Verification items for this drawing (mm, ordinates from the low corner). Give positions to 0.01 mm unless a question says otherwise; leave off trailing zeros. Order: outer loops, then holes, each group sorted by start corner. A loop starts at its lowest first (then second) coordinate and runs counter-clockwise, first axis right, second up.
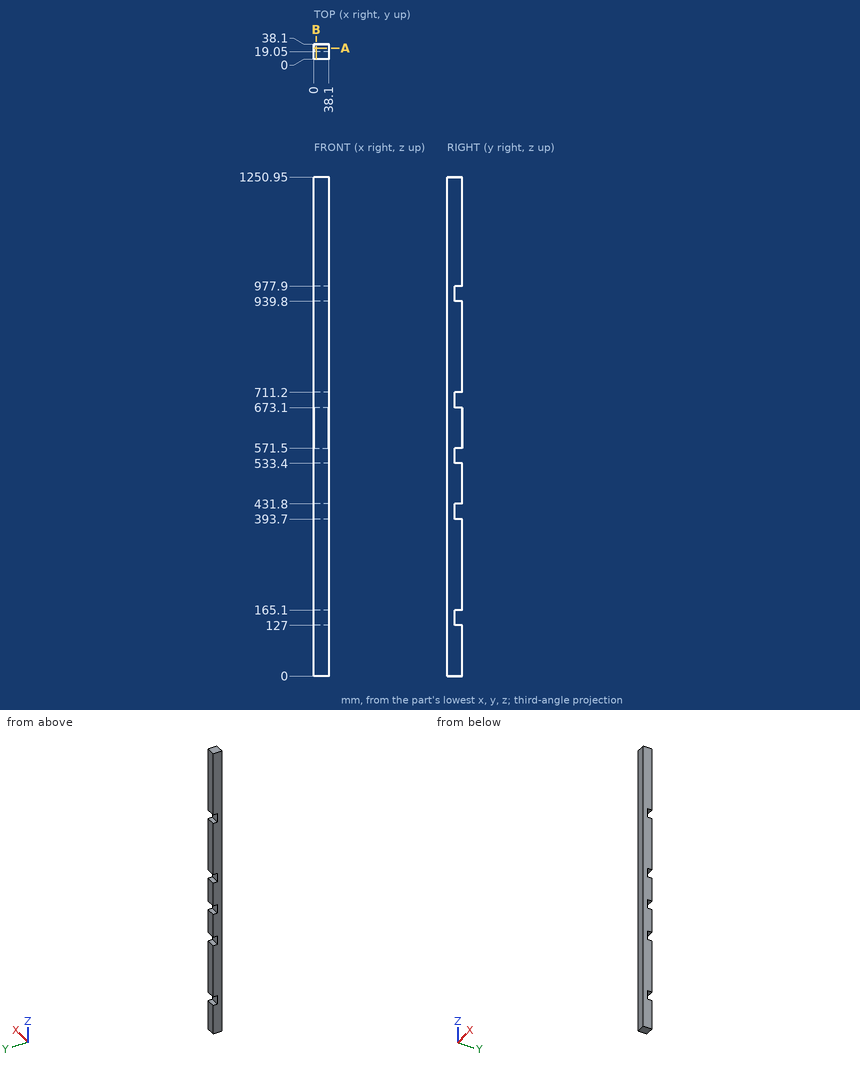
Q1. Cross-section at A-A, the plane y = 28. Record the boundary of the cut face in (x, z), and give its area (3 significant figures).
Q2. Cross-section at B-B, the plane x = 6. Record the boundary of the cut face in (y, z).
Q3. Gauge pin test, flat end, axial feed: P1, Ø11.5, axis at x = 26.5, z = 550.5, coming from the +Y side. Record the tip position at first contact, or that the pin passes through.
Q4. Thickness scan on L1, parallel to Z at x = 36, y = 21.5; L2, parallel to Y at x = 9, z = 970.5. Record the ranges inside material, lowest first.
Answers follow:
1. outline: (0, 0) - (38.1, 0) - (38.1, 127) - (0, 127) - close; (0, 165.1) - (38.1, 165.1) - (38.1, 393.7) - (0, 393.7) - close; (0, 431.8) - (38.1, 431.8) - (38.1, 533.4) - (0, 533.4) - close; (0, 571.5) - (38.1, 571.5) - (38.1, 673.1) - (0, 673.1) - close; (0, 711.2) - (38.1, 711.2) - (38.1, 939.8) - (0, 939.8) - close; (0, 977.9) - (38.1, 977.9) - (38.1, 1250.95) - (0, 1250.95) - close
1. area: 40,400 mm2
2. outline: (0, 0) - (38.1, 0) - (38.1, 127) - (19.05, 127) - (19.05, 165.1) - (38.1, 165.1) - (38.1, 393.7) - (19.05, 393.7) - (19.05, 431.8) - (38.1, 431.8) - (38.1, 533.4) - (19.05, 533.4) - (19.05, 571.5) - (38.1, 571.5) - (38.1, 673.1) - (19.05, 673.1) - (19.05, 711.2) - (38.1, 711.2) - (38.1, 939.8) - (19.05, 939.8) - (19.05, 977.9) - (38.1, 977.9) - (38.1, 1250.95) - (0, 1250.95) - close
3. P1: stops at y = 19.05
4. L1: z = 0 to 127, 165.1 to 393.7, 431.8 to 533.4, 571.5 to 673.1, 711.2 to 939.8, 977.9 to 1250.95
4. L2: y = 0 to 19.05
